```python
from build123d import *

# Parameters (mm, degrees)
F2_R     = 10
F3_DEPTH = 25
F2_R_2   = 15
F4_DEPTH = 5


with BuildPart() as f1:
    # F0 (on Front) → F1 (revolve)
    with BuildSketch(Plane.XZ):
        Polygon((7.5, 0), (-7.5, 0), (-7.5, -30), (-22.5, -30), (-22.5, -40), (7.5, -40), align=None)
    revolve(axis=Axis((0, 0, 0), (-1, 0, 0)))

    # F2 (on face) → F3 (cut)
    with BuildSketch(Plane.YZ.offset(7.5)):
        Circle(F2_R)
    extrude(amount=-F3_DEPTH, mode=Mode.SUBTRACT)

    # F2 (on face) → F4 (cut)
    with BuildSketch(Plane.YZ.offset(7.5)):
        Circle(F2_R_2)
        Circle(F2_R, mode=Mode.SUBTRACT)
    extrude(amount=-F4_DEPTH, mode=Mode.SUBTRACT)


solid = f1.part
```
Input: part model. Units: mm. Frame: model coordinates. A direction names the side the tool comes from. Give positions to 0.01 mm unless a question says otherwise; leave off trailing zeros. Order: outer loops, then holes, each group sorted by start corner. A loop starts at its lowest first (then second) coordinate and runs counter-clockwise, first axis right, second up.
1. Set-up query: faces 5 (the face through (7.5, -1, -17)), 6 (the face through (-7.5, 0, 13)), 7 (the face through (5.035, -14.985, 0.66)). Return all of +Z, -Z, +X, -X, +Y, -Y with unobstructed straight access to the full face (end or side cutting, diameter ignored); none if empty.
Computed:
face 5: +Z, -Z, +X, +Y, -Y
face 6: -X
face 7: +X
2. Draft query along Y for faces 1 (the face through (-7.29, 39.05, 8.67)), 2 (the face through (-2.43, -2.17, -9.76)), 3 (the face through (-22.5, -30, 6)), 4 (the face through (2.5, 3, -10)). Return one class per face: released by +Y, released by -Y, zero draft, split by the parting line, or undercut.
Computed:
face 1: split by the parting line
face 2: undercut
face 3: zero draft
face 4: undercut
3. Pin query (flat end, axial travel): pin 1 Ø10 at (x, z) = (-13.5, -14.5) entering from -Y; pin 2 Ø12 at (x, y) = (-1.5, 0.5) entering from +Z; pin 3 Ø3 at (x, y) = (-5.5, -24.5) entering from +Z; pin 4 Ø12 at (y, z) = (0, 0) entering from -X. Return the tip coordinate at first contact, or that it passes through.
Computed:
pin 1: stops at y = -38.86
pin 2: stops at z = 40
pin 3: stops at z = 32.73
pin 4: passes through
4. Line query: probe 1 along Z at (x, y) = (-13, 0); probe 2 along Z at (x, y) = (3.6, 0). Output: solid intervals per line, ascending.
Computed:
probe 1: z = -40 to -30, 30 to 40
probe 2: z = -40 to -15, 15 to 40
5. Cut plane A-A (y = 0). Return loops of the section in (x, z), and give its area (3 significant figures).
Computed:
outline: (-22.5, -40) - (7.5, -40) - (7.5, -15) - (2.5, -15) - (2.5, -10) - (-7.5, -10) - (-7.5, -30) - (-22.5, -30) - close; (-22.5, 30) - (-7.5, 30) - (-7.5, 10) - (2.5, 10) - (2.5, 15) - (7.5, 15) - (7.5, 40) - (-22.5, 40) - close
area: 1,150 mm2
6. Cut plane D-D (y = -26.5). Return loops of the section in (x, z), and give its area (3 significant figures).
Computed:
outline: (-22.5, -29.96) - (7.5, -29.96) - (7.5, 29.96) - (-22.5, 29.96) - (-22.5, 14.06) - (-7.5, 14.06) - (-7.5, -14.06) - (-22.5, -14.06) - close
area: 1,380 mm2
7. Cut plane C-C (x = -8.75). Return loops of the section in (y, z).
Computed:
outline: circle Ø80 at (0, 0); hole circle Ø60 at (0, 0)
